The drawing under review shows one solid part. Ordinate dimensions are in mm from its lowest x, y, z. A direction names the side the tool comes from. Coordinates: 2 decimals unless noted, no trailing zeros. Write each loop counter-clockwise with the first axis right and the second up, starting at its lowest first coordinate (ties: lowest second). Pieces come first, ordered by that corner, then holes.
Q1. Insertion check: pin 1 (5 mm diameter, centred on x = 10, y = 5, fed in from +Z); pin 2 (1 mm diameter, centred on x = 7.5, z = 7.5, fed in from +Y); pin 3 (4.5 mm diameter, centred on x = 16.5, z = 7.5, fed in from +Y). Each pin has a flat end and moves straight along its axis. Give the tip position at first contact, or say it passes through.
Q2. Take a section at B-B (z = 12.75). Give the boundary of the cut face in (x, y).
Q3. Machinability: for the marked faces 4, 5 and 6, which of the approach directions +Z, -Z, +X, -X, +Y, -Y give a long, thin tool a straight path to every point of the face, cutting with its end or side? Answer none if there is none.
Q4. Mouldability with a two-part tool opening along Y and no side actions: class the marked faces 1, 2 and 3 as pulls with the +Y half, pulls with the -Y half, needs draft (parallel to the pull), parting line crosses it, or undercut.
Q5. Take a section at D-D (x = 18). Give the boundary of the cut face in (y, z), and give its area (3 significant figures).
Q6. Take a section at A-A (y = 5). Give the boundary of the cut face in (x, z).
Q7. Take a section at C-C (x = 10). Give the boundary of the cut face in (y, z), and give its area (3 significant figures).
Q8. For probe 1 along Y at (x, z) = (10, 3.25); probe 2 along X at (y, z) = (5, 11); probe 3 along Z at (x, y) = (18, 7), list the stretches that pass through material, from the lowest coordinate up.
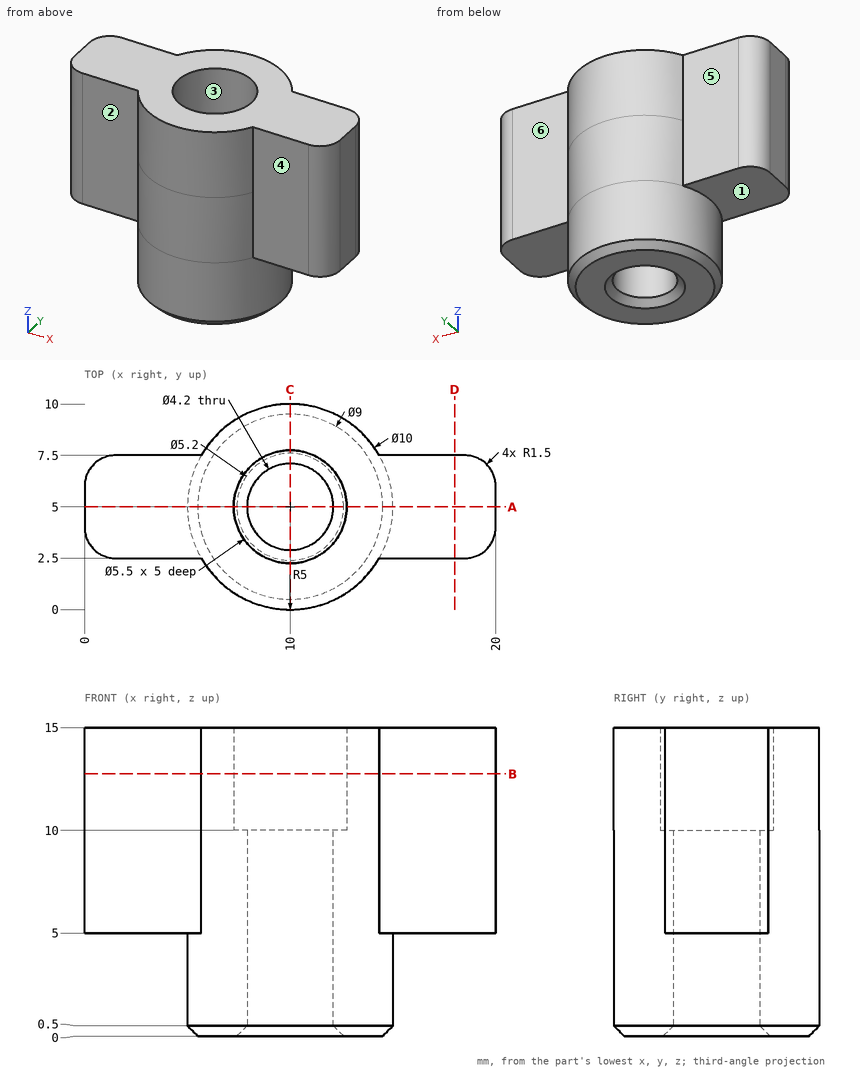
Response:
1. pin 1: stops at z = 10
1. pin 2: stops at y = 9.58
1. pin 3: stops at y = 7.63
2. outline: (0, 4) arc R1.5 ccw to (1.5, 2.5) - (5.67, 2.5) arc R5 ccw to (14.33, 2.5) - (18.5, 2.5) arc R1.5 ccw to (20, 4) - (20, 6) arc R1.5 ccw to (18.5, 7.5) - (14.33, 7.5) arc R5 ccw to (5.67, 7.5) - (1.5, 7.5) arc R1.5 ccw to (0, 6) - close; hole circle Ø5.5 at (10, 5)
3. face 4: +Z, -Z, +X, -Y
3. face 5: +Z, -Z, -X, +Y
3. face 6: +Z, -Z, +X, +Y
4. face 1: needs draft
4. face 2: pulls with the -Y half
4. face 3: undercut
5. outline: (2.5, 5) - (7.5, 5) - (7.5, 15) - (2.5, 15) - close
5. area: 50.0 mm2
6. outline: (0, 5) - (5, 5) - (5, 0.5) - (5.5, 0) - (7.4, 0) - (7.9, 0.5) - (7.9, 10) - (7.25, 10) - (7.25, 15) - (0, 15) - close; (12.1, 0.5) - (12.6, 0) - (14.5, 0) - (15, 0.5) - (15, 5) - (20, 5) - (20, 15) - (12.75, 15) - (12.75, 10) - (12.1, 10) - close
7. outline: (0, 0.5) - (0.5, 0) - (2.4, 0) - (2.9, 0.5) - (2.9, 10) - (2.25, 10) - (2.25, 15) - (0, 15) - close; (7.1, 0.5) - (7.6, 0) - (9.5, 0) - (10, 0.5) - (10, 15) - (7.75, 15) - (7.75, 10) - (7.1, 10) - close
7. area: 80.0 mm2
8. probe 1: y = 0 to 2.9, 7.1 to 10
8. probe 2: x = 0 to 7.25, 12.75 to 20
8. probe 3: z = 5 to 15
